Build history of the part. All positions in model axes, mm. A direction names the side the tool comes from. Round coordinates to 2 decimals unless told otherwise and drop trailing zeros. Write each loop counter-clockwise with the first axis right and the second up, starting at its lowest first coordinate (ties: lowest second). Pieces come first, ordered by that corner, then holes. Notation, with made-up numbers: (-20, 83) - (35, 83) arc R23 cw to (35, 107) - close; hole circle Ø3 at (74.5, 64.5). An arc over 180 degrees is marked (long way). Write each question's results on one line, items separated by ' | '.
from build123d import *

# Parameters (mm, degrees)
SKETCH_W     = 120
SKETCH_H     = 120
SKETCH_R     = 2.25
SKETCH_R_2   = 25
PAD_DEPTH    = 3
FILLET_R     = 2
CHAMFER_SIZE = 4
SKETCH001_R  = 2
POCKET_DEPTH = 3.001


with BuildPart() as part:
    # Sketch → Pad (new body)
    with BuildSketch(Plane.XY):
        Rectangle(SKETCH_W, SKETCH_H)
        with Locations((-55, 55)):
            Circle(SKETCH_R, mode=Mode.SUBTRACT)
        with Locations((55, 55)):
            Circle(SKETCH_R, mode=Mode.SUBTRACT)
        with Locations((55, -55)):
            Circle(SKETCH_R, mode=Mode.SUBTRACT)
        with Locations((-55, -55)):
            Circle(SKETCH_R, mode=Mode.SUBTRACT)
        Circle(SKETCH_R_2, mode=Mode.SUBTRACT)
    extrude(amount=PAD_DEPTH)

    # Fillet
    fillet_edges = [part.edges().sort_by_distance(p)[0] for p in [
        (-25, 0, 0),
    ]]
    fillet(fillet_edges, radius=FILLET_R)

    # Chamfer
    chamfer_edges = [part.edges().sort_by_distance(p)[0] for p in [
        (-60, -60, 1.5),
        (60, -60, 1.5),
        (60, 60, 1.5),
        (-60, 60, 1.5),
    ]]
    chamfer(chamfer_edges, length=CHAMFER_SIZE)

    # Sketch001 (on Face1 of Chamfer) → Pocket (cut, through all)
    with BuildSketch(Plane.XY.offset(3)):
        with Locations((0, 32.5)):
            Circle(SKETCH001_R)
        with Locations((32.5, 0)):
            Circle(SKETCH001_R)
        with Locations((0, -32.5)):
            Circle(SKETCH001_R)
        with Locations((-32.5, 0)):
            Circle(SKETCH001_R)
        with BuildLine():
            Line((-60, 47.5), (-33.835096, 21.335096))
            ThreePointArc((-33.835096, 21.335096), (-40, 0), (-33.835096, -21.335096))
            Line((-33.835096, -21.335096), (-60, -47.5))
            Line((-60, 47.5), (-60, -47.5))
        make_face()
        with BuildLine():
            Line((-47.5, -60), (-21.335096, -33.835096))
            ThreePointArc((-21.335096, -33.835096), (0, -40), (21.335096, -33.835096))
            Line((21.335096, -33.835096), (47.5, -60))
            Line((-47.5, -60), (47.5, -60))
        make_face()
        with BuildLine():
            Line((60, -47.5), (33.835096, -21.335096))
            ThreePointArc((33.835096, -21.335096), (40, 0), (33.835096, 21.335096))
            Line((33.835096, 21.335096), (60, 47.5))
            Line((60, -47.5), (60, 47.5))
        make_face()
        with BuildLine():
            Line((47.5, 60), (21.335096, 33.835096))
            ThreePointArc((21.335096, 33.835096), (0, 40), (-21.335096, 33.835096))
            Line((-21.335096, 33.835096), (-47.5, 60))
            Line((47.5, 60), (-47.5, 60))
        make_face()
    extrude(amount=-POCKET_DEPTH, mode=Mode.SUBTRACT)


solid = part.part
(1) Two-plate mould, pull along Y, no slides. Class faces 1 (the flat face through (52, 60, 1)), 2 (the flat face through (-34.6, -47.1, 1.5)), 3 (the flat face through (-60, 52, 1)), 4 (the cylindrical face through (-57.248, -54.901, 1.479)): released by +Y, released by -Y, zero draft, split by the parting line, or undercut.
Worked answers:
face 1: released by +Y | face 2: released by -Y | face 3: zero draft | face 4: undercut
(2) Flat gauge pins, fed straight in: pin 1 Ø2.5 at (x, y) = (32.5, 0) entering from +Z; pin 2 Ø1.5 at (y, z) = (-33, 1.5) entering from +X. Where does each tip first touch, or does it go through?
Worked answers:
pin 1: passes through | pin 2: stops at x = 46.25
(3) Tool access for faces 5 (the cylindrical face through (52.752, -54.901, 1.479)), 6 (the flat face through (-34.2, 46.7, 1.5)), 7 (the flat face through (34.2, -46.7, 1.5)), 8 (the flat face through (46.7, 34.2, 1.5)): list every direction of +Z, -Z, +X, -X, +Y, -Y with a clear straight run to the whole face (end or side of a thin tool).
Worked answers:
face 5: +Z, -Z | face 6: +Z, -Z, +Y | face 7: +Z, -Z, -Y | face 8: +Z, -Z, +X
(4) Slice it at A-A, the plane y = 0. Write the cut outline in (x, z), and give its area (3 significant figures).
Worked answers:
outline: (-40, 0) - (-34.5, 0) - (-34.5, 3) - (-40, 3) - close; (-30.5, 0) - (-27, 0) arc R2 ccw to (-25, 2) - (-25, 3) - (-30.5, 3) - close; (25, 2) arc R2 ccw to (27, 0) - (30.5, 0) - (30.5, 3) - (25, 3) - close; (34.5, 0) - (40, 0) - (40, 3) - (34.5, 3) - close | area: 64.3 mm2
(5) Slice it at C-C, the plane y = 37.5. Write the cut outline in (x, z).
Worked answers:
outline: (-50, 0) - (-25, 0) - (-25, 3) - (-50, 3) - close; (-13.92, 0) - (13.92, 0) - (13.92, 3) - (-13.92, 3) - close; (25, 0) - (50, 0) - (50, 3) - (25, 3) - close
(6) Slice it at B-B, the plane z = 1. State how many separate pieces and enclosed holes the cut face has, and give its area (3 significant figures).
Worked answers:
separate pieces: 1 | enclosed holes: 9 | area: 5,760 mm2
(7) Drill centre lines: probe 1 along Y at (x, z) = (55, 0.7); probe 2 along Y at (x, z) = (0, 1); probe 3 along X at (y, z) = (48, 1.05). Where is each one in solid material? Low to high. Write a range as [from, to].
Worked answers:
probe 1: y = [-60, -57.25], [-52.75, -42.5], [42.5, 52.75], [57.25, 60] | probe 2: y = [-40, -34.5], [-30.5, -25.27], [25.27, 30.5], [34.5, 40] | probe 3: x = [-60, -35.5], [35.5, 60]
